Here's how the part is built. I have some questions about the finished solid (model axes, mm). A direction names the side the tool comes from. Round coordinates to 2 decimals unless told otherwise and drop trailing zeros. Loops run counter-clockwise (first coordinate to the right, second up) from the corner with the lowest first, then second, coordinate; pieces in that order, holes last. Notation, with made-up numbers: (13.5, -31) - (59.5, -31) arc R25 ccw to (59.5, 2) - close; hole circle Ø4 at (86, 35.25). An arc over 180 degrees is marked (long way). Answer as a JSON object with one key per item and string values. Group by question number.
1) I want a section at B-B, the plane z = 8. Please give me the cut outline in (x, y), then the cut area to 3 significant figures.
2) Which directions (+Z, -Z, +X, -X, +Y, -Y) give clear straight access to the entire face, cutting with the end or side of a thin tool? Please do faces 3 (the face through (8, 42, 9)), 4 (the face through (-4.88, 42.99, -1.08)), 5 (the face through (-29.35, 20.71, 32.13)).
3) I want a section at C-C, the plane x = -10.5. Please give me the cut outline in (y, z), then the cut area to 3 significant figures.
4) I want a section at D-D, the plane y = 22. Give the number of separate pieces and of enclosed holes in the cut face, then the cut area to 3 significant figures.
5) Will these pins go through, and if not, where does the flat tip stop? P1, Ø10, axis at y = 19, z = 18.5, coming from the -X side; P2, Ø10, axis at x = 2, y = 25, coming from the -Z side; P3, Ø5, axis at x = 33.5, z = 11.5, coming from the -Y side; P4, Ø3, axis at y = 16.5, z = -11.5, coming from the +X side.
6) If we mould it in two halves opening along X, with no side actions, what happens to faces 1 (the face through (13, 0, -41)), 2 (the face through (-36, 36, 4))? For each: pulls with the +X half, pulls with the -X half, needs draft (parallel to the pull), parting line crosses it, or undercut.
7) I want a section at A-A, the plane y = 10. Please give me the cut outline in (x, z), then the cut area to 3 significant figures.
8) If I drill on line 1 along X through (y, z) = (3.5, 0); line 2 along X through (y, z) = (43, 0); line 3 along Y through (x, z) = (-7, 28.5), over which ranges is the centre line in solid material (lowest first)? Write a range as [from, to].
from build123d import *

# Parameters (mm, degrees)
AUFSATZ_LINEAR_AUSTRAGEN1_DEPTH = 44
AUFSATZ_LINEAR_START            = -2
SKIZZE2_R                       = 45
SKIZZE2_R_2                     = 5
AUFSATZ_LINEAR_AUSTRAGEN2_DEPTH = 2
SKIZZE3_R                       = 8
SCHNITT_LINEAR_AUSTRAGEN2_DEPTH = 9.26
AUFSATZ_LINEAR_AUSTRAGEN3_DEPTH = 4
KREISMUSTER1_COUNT              = 3
KREISMUSTER1_ANGLE              = 180


with BuildPart() as part:
    # Skizze1 → Aufsatz-Linear austragen1 (new body)
    with BuildSketch(Plane(origin=(0, 0, 0), x_dir=(1, 0, 0), z_dir=(0, 1, 0))):
        with BuildLine():
            Line((28.22984402, -31.097844083), (29.932068323, -33.601655999))
            ThreePointArc((29.932068323, -33.601655999), (0.280437371, 44.999126157), (-30.348542355, -33.225983461))
            Line((-30.348542355, -33.225983461), (-28.325306198, -31.010917897))
            ThreePointArc((-28.325306198, -31.010917897), (0.064554608, 41.999950389), (28.22984402, -31.097844083))
        make_face()
    extrude(amount=AUFSATZ_LINEAR_AUSTRAGEN1_DEPTH)

    # Skizze2 → Aufsatz-Linear austragen2 (add)
    with BuildSketch(Plane(origin=(0, 44, 0), x_dir=(1, 0, 0), z_dir=(0, 1, 0)).offset(AUFSATZ_LINEAR_START)):
        with Locations(Location((0, 0, 0), (0, 0, 227.591490679))):
            Circle(SKIZZE2_R)
        with Locations(Location((0, 0, 0), (0, 0, 270))):
            Circle(SKIZZE2_R_2, mode=Mode.SUBTRACT)
    extrude(amount=AUFSATZ_LINEAR_AUSTRAGEN2_DEPTH)

    # Skizze3 → Schnitt-Linear austragen2 (cut)
    with BuildSketch(Plane(origin=(0, 0, -45), x_dir=(-1, 0, 0), z_dir=(0, 0, -1))):
        with Locations((0, 11.392175051)):
            Circle(SKIZZE3_R)
    extrude(amount=-SCHNITT_LINEAR_AUSTRAGEN2_DEPTH, mode=Mode.SUBTRACT)

    # Skizze4 → Aufsatz-Linear austragen3 (add, symmetric)
    with BuildSketch(Plane.XY):
        with BuildLine():
            Line((-41.880766109, 42), (-41.880766109, 19.345066602))
            add(Edge.make_bspline(
                [(-41.880766109, 19.345066602), (-37.634088063, 37.128030919), (-19.638651498, 42)],
                knots=[0, 0, 0, 1, 1, 1], degree=2))
            Line((-19.638651498, 42), (-41.880766109, 42))
        make_face()
    aufsatz_linear_austragen3 = extrude(amount=AUFSATZ_LINEAR_AUSTRAGEN3_DEPTH, both=True)

    # Kreismuster1: Aufsatz-Linear austragen3 ×3 about axis
    kreismuster1_axis = Axis((0, 42, 0), (0, -1, 0))
    for i in range(1, KREISMUSTER1_COUNT):
        add(aufsatz_linear_austragen3.rotate(kreismuster1_axis, i * KREISMUSTER1_ANGLE / (KREISMUSTER1_COUNT - 1)))


solid = part.part
Outcome:
{
 "1": {"outline": "(-44.28, 0) - (-41.23, 0) - (-41.23, 42) - (41.23, 42) - (41.23, 0) - (44.28, 0) - (44.28, 44) - (-44.28, 44) - close", "area": "434 mm^2"},
 "2": {"face 3": "-Y", "face 4": "+Y, -Y", "face 5": "+Z, -Y"},
 "3": {"outline": "(0, -43.76) - (44, -43.76) - (44, 43.76) - (42, 43.76) - (42, -40.67) - (0, -40.67) - close", "area": "305 mm^2"},
 "4": {"separate pieces": "1", "enclosed holes": "3", "area": "645 mm^2"},
 "5": {"P1": "x = -42.93", "P2": "z = -45", "P3": "y = 42", "P4": "x = 43.87"},
 "6": {"face 1": "needs draft", "face 2": "undercut"},
 "7": {"outline": "(-30.35, 33.23) arc R45 ccw to (-7.88, -44.31) - (-7.88, -41.25) arc R42 cw to (-28.33, 31.01) - close; (7.88, -44.31) arc R45 ccw to (29.93, 33.6) - (28.23, 31.1) arc R42 cw to (7.88, -41.25) - close", "area": "580 mm^2"},
 "8": {"line 1": "[-45, -42], [42, 45]", "line 2": "[-45, -5], [5, 45]", "line 3": "[42, 44]"}
}
